Source: CAD feature listing. Evaluate the final solid. Frame: model axes, mm. A direction names the side the tool comes from. Coordinates: 2 decimals unless noted, no trailing zeros. Order: outer loops, then holes, each group sorted by start corner. A loop starts at its lowest first (then second) coordinate and runs counter-clockwise, first axis right, second up. Notation, with made-up numbers: (55.5, 68.25) -> (108.5, 68.25) arc R13 cw to (108.5, 91.25) -> close; hole circle Ø1 at (4.25, 20.5). An arc over 180 degrees is marked (long way). Write each question's results on one line, items separated by ' | '. Start each with the question number.
from build123d import *

# Parameters (mm, degrees)
SKETCH083_W     = 244
SKETCH083_H     = 244
PAD053_DEPTH    = 1.6
SKETCH084_W     = 12.805552
SKETCH084_H     = 4.986233
SKETCH084_W_2   = 11.219025
SKETCH084_H_2   = 6.742746
SKETCH084_W_3   = 10.085793
SKETCH084_H_3   = 3.059733
SKETCH084_W_4   = 10.482422
SKETCH084_H_4   = 3.003072
SKETCH084_W_5   = 25.894417
SKETCH084_H_5   = 5.099556
SKETCH084_W_6   = 13.772156
SKETCH084_H_6   = 4.775269
SKETCH084_W_7   = 24.776046
SKETCH084_H_7   = 5.121302
SKETCH084_W_8   = 11.765168
SKETCH084_H_8   = 2.906684
SKETCH084_W_9   = 7.128295
SKETCH084_H_9   = 11.142288
SKETCH084_W_10  = 10.311813
SKETCH084_H_10  = 2.837479
SKETCH084_W_11  = 10.311814
SKETCH084_H_11  = 2.837478
SKETCH084_W_12  = 7.015946
SKETCH084_H_12  = 11.242416
SKETCH084_W_13  = 11.016556
SKETCH084_H_13  = 6.50441
PAD054_DEPTH    = 10
SKETCH085_W     = 15.253067
SKETCH085_H     = 33.165085
SKETCH085_W_2   = 7.187866
SKETCH085_H_2   = 23.70736
SKETCH085_W_3   = 5.42244
SKETCH085_H_3   = 12.736404
SKETCH085_W_4   = 12.425812
SKETCH085_H_4   = 5.750149
SKETCH085_W_5   = 4.511801
SKETCH085_H_5   = 8.449646
PAD055_DEPTH    = 15
SKETCH086_W     = 10.737412
SKETCH086_H     = 53.687088
SKETCH086_W_2   = 31.147434
SKETCH086_H_2   = 11.349274
PAD056_DEPTH    = 20
SKETCH089_W     = 90
SKETCH089_H     = 9.5
PAD059_DEPTH    = 11
SKETCH090_W     = 81.9
SKETCH090_H     = 22
PAD061_DEPTH    = 6
SKETCH100_R     = 1.7
HOLE_DEPTH      = 1.601
SKETCH_W        = 69
SKETCH_H        = 12
SKETCH_W_2      = 12
SKETCH_H_2      = 69
PAD_DEPTH       = 12
SKETCH116_W     = 11.2
SKETCH116_H     = 1.6
SKETCH116_W_2   = 71.15
POCKET029_DEPTH = 7.35


with BuildPart() as part:
    # Sketch083 → Pad053 (new body)
    with BuildSketch(Plane.XY):
        with Locations((122, 122)):
            Rectangle(SKETCH083_W, SKETCH083_H)
    extrude(amount=PAD053_DEPTH)

    # Sketch084 (on Face6 of Pad053) → Pad054 (join)
    with BuildSketch(Plane.XY.offset(1.6)):
        with Locations((25.66175, 8.1425655)):
            Rectangle(SKETCH084_W, SKETCH084_H)
        with Locations((60.3814395, 7.038229)):
            Rectangle(SKETCH084_W_2, SKETCH084_H_2)
        with Locations((82.4398765, 7.0638115)):
            Rectangle(SKETCH084_W_3, SKETCH084_H_3)
        with Locations((101.593994, 6.977586)):
            Rectangle(SKETCH084_W_4, SKETCH084_H_4)
        with Locations((125.3647115, 8.201877)):
            Rectangle(SKETCH084_W_5, SKETCH084_H_5)
        with Locations((176.093216, 7.6274735)):
            Rectangle(SKETCH084_W_6, SKETCH084_H_6)
        with Locations((225.320961, 8.494646)):
            Rectangle(SKETCH084_W_7, SKETCH084_H_7)
        with Locations((203.897812, 15.63834)):
            Rectangle(SKETCH084_W_8, SKETCH084_H_8)
        with Locations((222.3003845, 162.861565)):
            Rectangle(SKETCH084_W_9, SKETCH084_H_9)
        with Locations((226.3459395, 237.2302015)):
            Rectangle(SKETCH084_W_10, SKETCH084_H_10)
        with Locations((226.276741, 230.032692)):
            Rectangle(SKETCH084_W_11, SKETCH084_H_11)
        with Locations((165.498787, 226.013008)):
            Rectangle(SKETCH084_W_12, SKETCH084_H_12)
        with Locations((50.544289, 227.792839)):
            Rectangle(SKETCH084_W_13, SKETCH084_H_13)
    extrude(amount=PAD054_DEPTH)

    # Sketch085 (on Face5 of Pad054) → Pad055 (join)
    with BuildSketch(Plane.XY.offset(1.6)):
        with Locations((236.3734665, 41.3033025)):
            Rectangle(SKETCH085_W, SKETCH085_H)
        with Locations((236.016449, 109.243)):
            Rectangle(SKETCH085_W_2, SKETCH085_H_2)
        with Locations((234.125511, 136.078026)):
            Rectangle(SKETCH085_W_3, SKETCH085_H_3)
        with Locations((228.421982, 21.4103315)):
            Rectangle(SKETCH085_W_4, SKETCH085_H_4)
        with Locations((237.1440995, 20.060583)):
            Rectangle(SKETCH085_W_5, SKETCH085_H_5)
    extrude(amount=PAD055_DEPTH)

    # Sketch086 (on Face5 of Pad055) → Pad056 (join)
    with BuildSketch(Plane.XY.offset(1.6)):
        with Locations((234.692436, 180.943504)):
            Rectangle(SKETCH086_W, SKETCH086_H)
        with Locations((54.290396, 236.828354)):
            Rectangle(SKETCH086_W_2, SKETCH086_H_2)
    extrude(amount=PAD056_DEPTH)

    # Sketch089 → Pad059 (join)
    with BuildSketch(Plane.XY.offset(1.6)):
        with Locations((87.75, 19.75)):
            Rectangle(SKETCH089_W, SKETCH089_H)
    extrude(amount=PAD059_DEPTH)

    # Sketch090 (on Face5 of Pad059) → Pad061 (join)
    with BuildSketch(Plane.XY.offset(1.6)):
        with Locations((105.95, 39.5)):
            Rectangle(SKETCH090_W, SKETCH090_H)
    extrude(amount=PAD061_DEPTH)

    # Sketch100 → Hole (cut, through all)
    with BuildSketch(Plane.XY.offset(1.6)):
        with Locations((82.56, 123)):
            Circle(SKETCH100_R)
        with Locations((160.56, 123)):
            Circle(SKETCH100_R)
        with Locations((160.56, 201)):
            Circle(SKETCH100_R)
        with Locations((82.56, 201)):
            Circle(SKETCH100_R)
        with Locations((33.02, 237.83)):
            Circle(SKETCH100_R)
        with Locations((165.1, 237.83)):
            Circle(SKETCH100_R)
        with Locations((237.49, 237.83)):
            Circle(SKETCH100_R)
        with Locations((237.49, 80.35)):
            Circle(SKETCH100_R)
        with Locations((165.1, 80.35)):
            Circle(SKETCH100_R)
        with Locations((165.1, 14.31)):
            Circle(SKETCH100_R)
        with Locations((10.16, 34.63)):
            Circle(SKETCH100_R)
        with Locations((10.16, 80.35)):
            Circle(SKETCH100_R)
    extrude(amount=-HOLE_DEPTH, mode=Mode.SUBTRACT)

    # Sketch (on Face5 of Pad061) → Pad (join)
    with BuildSketch(Plane.XY.offset(1.6)):
        with Locations((112.5, 217.5)):
            Rectangle(SKETCH_W, SKETCH_H)
        with Locations((68, 166.75)):
            Rectangle(SKETCH_W_2, SKETCH_H_2)
    extrude(amount=PAD_DEPTH)

    # Sketch116 (on Face119 of Pad) → Pocket029 (cut)
    with BuildSketch(Plane.XY.offset(12.6)):
        with Locations((51.25, 19.75)):
            Rectangle(SKETCH116_W, SKETCH116_H)
        with Locations((94.275, 19.75)):
            Rectangle(SKETCH116_W_2, SKETCH116_H)
    extrude(amount=-POCKET029_DEPTH, mode=Mode.SUBTRACT)


solid = part.part
(1) Draft query along X for faces 5 (the flat face through (38.717, 237, 11)), 6 (the flat face through (54.772, 7, 7)), 7 (the flat face through (218.736, 163, 7)), 8 (the flat face through (235, 207.787, 11)). Return one class per face: released by +X, released by -X, zero draft, split by the parting line, or undercut.
(2) Section C-C on y = 182. Return the cut outline in (x, z), then the cut area to 3 significant figures.
(3) Line query: L1, parallel to Y at x = 133, z = 6.75; L2, parallel to Y at x = 82.56, z = 0.5; L3, parallel to Y at x = 165.1, z = 0.95. Output: solid intervals per line, ascending.
(4) Reachability of faces 1 (the flat face through (87, 21, 12.6)), 2 (the flat face through (222, 168.433, 7)), 3 (the flat face through (236, 97.389, 9)), 4 (the flat face through (112, 223.5, 8)) from +Z, -Z, +X, -X, +Y, -Y: full face, straight path, thin tool, end or side. Return the list, or none.
(5) First-contact query: P1, Ø8, axis at x = 202.5, y = 43, coming from the +Z side; P2, Ø1.5, axis at y = 9, z = 6, coming from the -X side; P3, Ø2, axis at y = 165, z = 10.5, coming from the +X side; P4, Ø2.5, axis at x = 160.56, y = 123, coming from the +Z side. Flat tips, straight axial feed; report the tip coordinate or a pass-through.
(6) Section B-B on x = 189.5. Return the cut outline in (y, z), then the cut area to 3 significant figures.
(7) Section A-A on y = 42.5. Return the cut outline in (x, z), then the cut area to 3 significant figures.
Results list:
1) face 5: released by -X | face 6: undercut | face 7: undercut | face 8: zero draft
2) outline: (0, 0) -> (244, 0) -> (244, 1.6) -> (240.06, 1.6) -> (240.06, 21.6) -> (229.32, 21.6) -> (229.32, 1.6) -> (74, 1.6) -> (74, 13.6) -> (62, 13.6) -> (62, 1.6) -> (0, 1.6) -> close | area: 749 mm²
3) L1: y = 5.65 to 10.75, 28.5 to 50.5, 211.5 to 223.5 | L2: y = 0 to 121.3, 124.7 to 199.3, 202.7 to 244 | L3: y = 0 to 12.61, 16.01 to 78.65, 82.05 to 236.13, 239.53 to 244
4) face 1: +Z, -X, -Y | face 2: +Z | face 3: +Z, +X, -X | face 4: +Z, -X, +Y
5) P1: stops at z = 1.6 | P2: stops at x = 19.26 | P3: stops at x = 240.06 | P4: passes through
6) outline: (0, 0) -> (244, 0) -> (244, 1.6) -> (0, 1.6) -> close | area: 390 mm²
7) outline: (0, 0) -> (244, 0) -> (244, 16.6) -> (228.75, 16.6) -> (228.75, 1.6) -> (146.9, 1.6) -> (146.9, 7.6) -> (65, 7.6) -> (65, 1.6) -> (0, 1.6) -> close | area: 1,110 mm²
